Input: dimensioned drawing with shaded views. Units: mm. Origin: part minimum x, y, z. Round coordinates to 2 decimals unless told otherwise and drop trailing zeros. Order: outer loops, then holes, each group sorted by start corner. A loop starts at its lowest first (then second) coordinate and runs counter-clockwise, first axis right, second up. Notation, with made-up numbers: (-24, -2.75) -> (14, -2.75) arc R22 ccw to (14, 28.25) -> close; hole circle Ø4 at (68, 38.5). An arc over 180 degrees is marked (long way). Use a Markdown table: item, result. Add a question column.
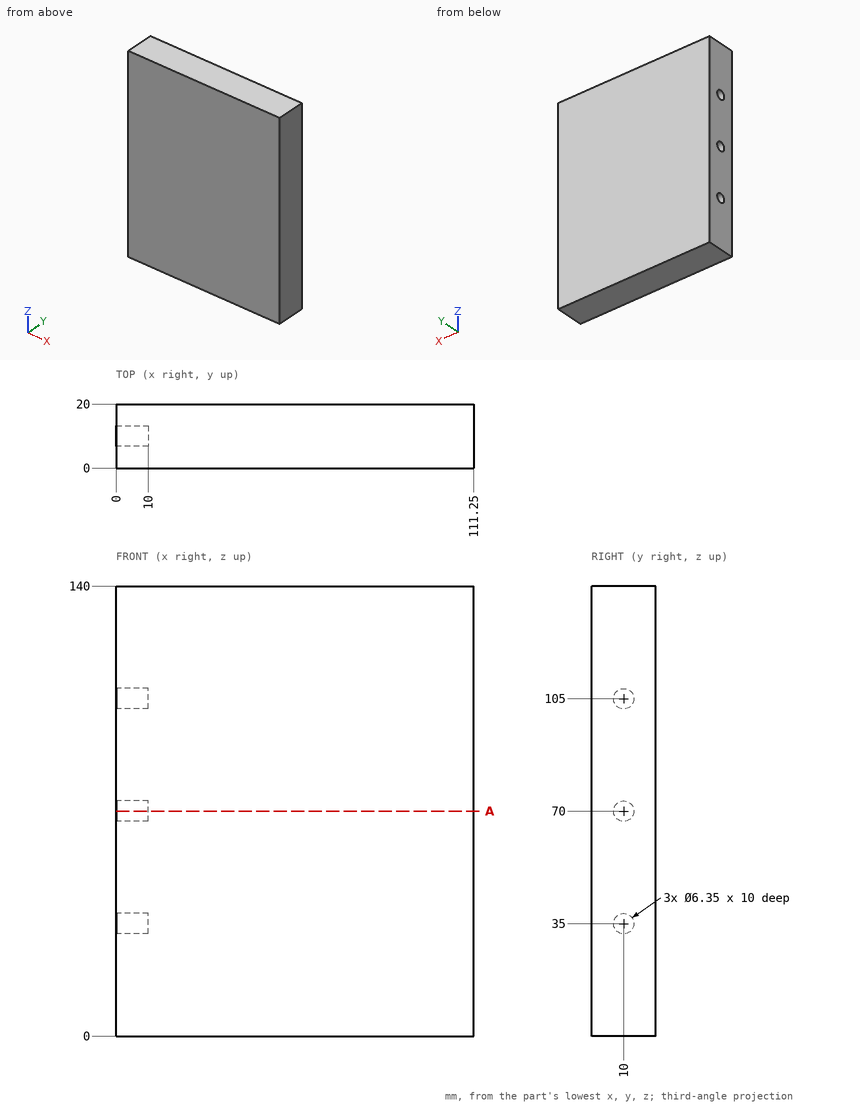
1) First-contact query: pin 1 Ø1.9 at (y, z) = (10, 34) entering from -X; pin 2 Ø10 at (y, z) = (10, 105) entering from -X. Flat tips, straight axial feed; report the tip coordinate or a pass-through.
2) Line query: probe 1 along Z at (x, y) = (8, 10) (3 decimals); probe 2 along Y at (x, z) = (6, 70) (3 decimals). Output: solid intervals per line, ascending. Write a range as from..to.
3) Section A-A on z = 70. Output: boundary loops of the cut face in (x, y) (3 decimals), then the cut area to 3 significant figures.
Conclusion:
| question | item | result |
|---|---|---|
| 1 | pin 1 | stops at x = 10 |
| 1 | pin 2 | stops at x = 0 |
| 2 | probe 1 | z = 0..31.825, 38.175..66.825, 73.175..101.825, 108.175..140 |
| 2 | probe 2 | y = 0..6.825, 13.175..20 |
| 3 | outline | (0, 0) -> (111.25, 0) -> (111.25, 20) -> (0, 20) -> (0, 13.175) -> (10, 13.175) -> (10, 6.825) -> (0, 6.825) -> close |
| 3 | area | 2,160 mm^2 |
